Design review of the part shown in the three views and the two pictorial views. Dimensions are in mm from the part's minimum x, y and z. A direction names the side the tool comes from. Coordinates: 2 decimals unless noted, no trailing zeros. Loops run counter-clockwise (first coordinate to the right, second up) from the corner with the lowest first, then second, coordinate; pieces in that order, holes last. Notation, with made-up numbers: M 56.5,-24 L 80.5,-24 A11 cw 80.5,-8 Z; hole C 53,64 d4. An arc over 180 degrees is marked long. Answer as a JSON object with one key per item and string values. Group by question number.
Item 1: Add section D-D (z = 3.75). State the section outline as (x, y) points.
Item 2: Add section B-B (y = 4.75). State the section outline as (x, z) points.
Item 3: Tool access review of the marked faces 1, 2 and 3: name each direction out of +Z, -Z, +X, -X, +Y, -Y from which nothing blocks a thin tool from reaching the whole face with its end or side.
Item 4: Add section A-A (x = 14). State the section outline as (y, z) points, then the cut area to 3 significant figures.
Item 5: Add section C-C (z = 9.75). State the section outline as (x, y) points.
Item 6: Wall thickness on L1, parallel to Y at x = 29.5, z = 20.25; L2, parallel to X at y = 4.25, z = 25.75; L3, parallel to Z at x = 16.5, y = 1.5: over which ranges is each line inside the solid? List them lowest first. Write a range as from..to.
Item 7: Insertion check: pin 1 (1 mm diameter, centred on x = 27.5, z = 12, fed in from -Y); pin 2 (0.6 mm diameter, centred on y = 1, z = 26.5, fed in from +X); pin 3 (0.6 mm diameter, centred on y = 0.5, z = 28, fed in from -X). Each pin has a flat end and moves straight along its axis. Give the tip position at first contact, or say it passes through.
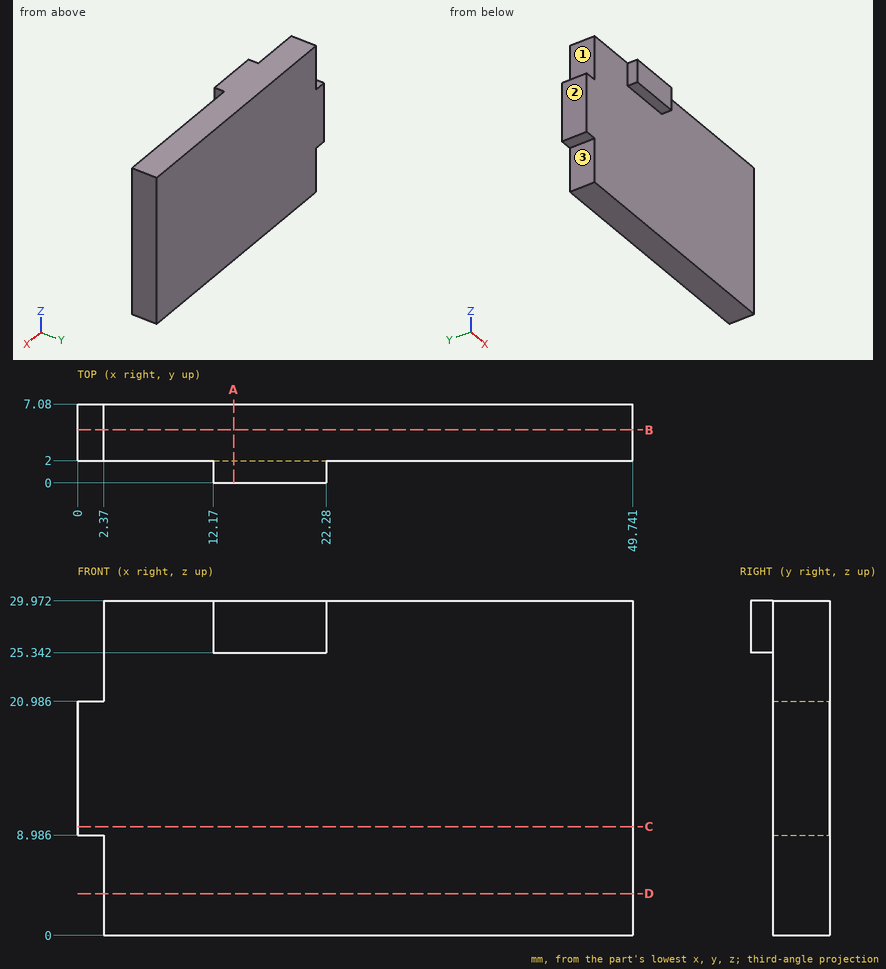
From the geometry:
{
 "1": {"outline": "M 2.37,2 L 49.74,2 L 49.74,7.08 L 2.37,7.08 Z"},
 "2": {"outline": "M 0,8.99 L 2.37,8.99 L 2.37,0 L 49.74,0 L 49.74,29.97 L 2.37,29.97 L 2.37,20.99 L 0,20.99 Z"},
 "3": {"face 1": "+Z, -X, +Y, -Y", "face 2": "+Z, -Z, -X, +Y, -Y", "face 3": "-Z, -X, +Y, -Y"},
 "4": {"outline": "M 0,25.34 L 2,25.34 L 2,0 L 7.08,0 L 7.08,29.97 L 0,29.97 Z", "area": "162 mm²"},
 "5": {"outline": "M 0,2 L 49.74,2 L 49.74,7.08 L 0,7.08 Z"},
 "6": {"L1": "y = 2..7.08", "L2": "x = 2.37..49.74", "L3": "z = 25.34..29.97"},
 "7": {"pin 1": "stops at y = 2", "pin 2": "stops at x = 22.28", "pin 3": "stops at x = 12.17"}
}
